Input: dimensioned drawing with shaded views. Units: mm. Origin: part minimum x, y, z. A direction names the side the tool comes from. Round coordinates to 2 decimals unless told otherwise and drop trailing zeros. Loops run counter-clockwise (first coordinate to the right, second up) from the corner with the lowest first, then second, coordinate; pieces in that order, holes last. Notation, with made-up numbers: (72, 88) - (103, 88) arc R23 cw to (103, 125) - close; hole circle Ø6 at (21.25, 45.5). An arc over 180 degrees is marked (long way). Answer as a JSON object with one key per item and string values. Group by question number.
Item 1: Section B-B (z = 6.25). Return the cut outline in (x, y) (1 decimal).
Item 2: Section D-D (y = 35). Return the cut outline in (x, z) (1 decimal).
Item 3: Section A-A (y = 22.5). Return the cut outline in (x, z), plus the area to 3 significant figures.
Item 4: Reachability of the marked faces 4, 5 and 6 from +Z, -Z, +X, -X, +Y, -Y: full face, straight path, thin tool, end or side. Return the list, or none.
Item 5: First-contact query: pin 1 (2 mm diameter, centred on y = 11.5, z = 16.5, fed in from -X); pin 2 (12 mm diameter, centred on x = 18.5, y = 23.5, fed in from -Z); pin 3 (6 mm diameter, centred on y = 16, z = 20.5, fed in from +X); pin 4 (0.6 mm diameter, centred on x = 44.5, y = 21, fed in from -Z). Flat tips, straight axial feed; report the tip coordinate or a pass-through.
Item 6: Section C-C (x = 12.5). Return the cut outline in (y, z).
Item 7: Line query: line 1 (X direction, y = 28, z = 13.75); line 2 (X direction, y = 20.5, z = 19.75); line 3 (Y direction, x = 5, z = 3.75) (1 decimal). Output: solid intervals per line, ascending.
Item 8: Draft query along X for the marked faces 1, 2 and 3. Return one class per face: released by +X, released by -X, zero draft, split by the parting line, or undercut.
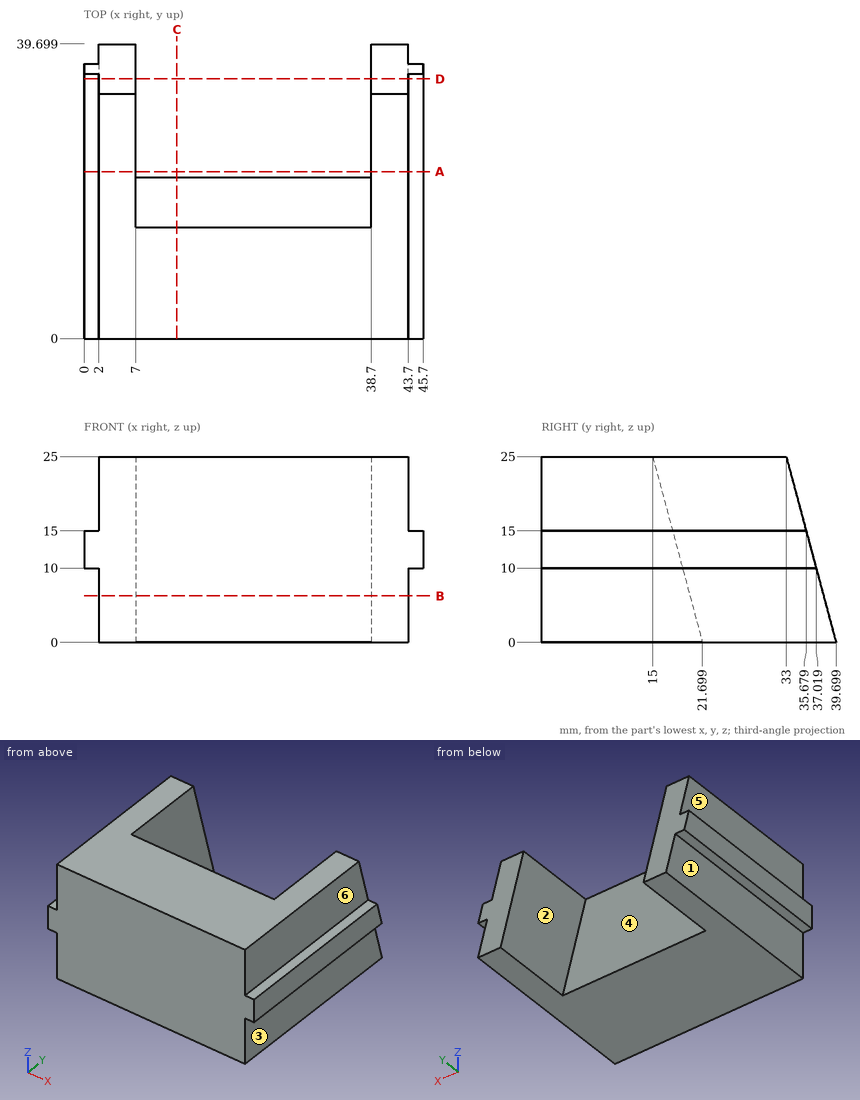
Values:
{
 "1": {"outline": "(2, 0) - (43.7, 0) - (43.7, 38) - (38.7, 38) - (38.7, 20) - (7, 20) - (7, 38) - (2, 38) - close"},
 "2": {"outline": "(0, 10) - (2, 10) - (2, 0) - (7, 0) - (7, 17.5) - (2, 17.5) - (2, 15) - (0, 15) - close; (38.7, 0) - (43.7, 0) - (43.7, 10) - (45.7, 10) - (45.7, 15) - (43.7, 15) - (43.7, 17.5) - (38.7, 17.5) - close"},
 "3": {"outline": "(0, 10) - (2, 10) - (2, 0) - (7, 0) - (7, 25) - (2, 25) - (2, 15) - (0, 15) - close; (38.7, 0) - (43.7, 0) - (43.7, 10) - (45.7, 10) - (45.7, 15) - (43.7, 15) - (43.7, 25) - (38.7, 25) - close", "area": "270 mm^2"},
 "4": {"face 4": "+Z, +Y", "face 5": "+Z, -X, +Y, -Y", "face 6": "+Z, +X, +Y, -Y"},
 "5": {"pin 1": "stops at x = 2", "pin 2": "stops at z = 0", "pin 3": "stops at x = 43.7", "pin 4": "stops at z = 10"},
 "6": {"outline": "(0, 0) - (21.7, 0) - (15, 25) - (0, 25) - close"},
 "7": {"line 1": "x = 0 to 7, 38.7 to 45.7", "line 2": "x = 2 to 7, 38.7 to 43.7", "line 3": "y = 0 to 38.7"},
 "8": {"face 1": "released by -X", "face 2": "undercut", "face 3": "released by +X"}
}
